Input: part model. Units: mm. Frame: model coordinates. Face numbers are marked on the shaded views. A direction names the side the tool comes from. Give positions to 0.01 mm unless a question says otherwise; leave off trailing zeros. Order: outer loops, then holes, each group sorted by start corner. A loop starts at its lowest first (then second) coordinate and runs counter-clockwise, first axis right, second up. Notation, with made-up numbers: M -32,58 L -12,58 A27 cw -12,90 Z; hole C -11,68 d2. An arc over 180 degrees is marked long. Use a Markdown table: item, result.
from build123d import *

# Parameters (mm, degrees)
CUT_EXTRUDE_1_DEPTH = 3.5


with BuildPart() as part:
    # 草图1 → 旋转1 (revolve)
    with BuildSketch(Plane.XY, mode=Mode.PRIVATE) as revolve_1_sk:
        with BuildLine():
            Line((-108.930747922, 0), (-108.930747922, 13))
            Line((-108.930747922, 13), (-106.930747922, 15))
            Line((-106.930747922, 15), (-80.930747922, 15))
            Line((-80.930747922, 15), (-80.930747922, 20))
            Line((-80.930747922, 20), (-71.930747922, 20))
            Line((-71.930747922, 20), (-71.930747922, 24))
            Line((-71.930747922, 24), (-69.930747922, 26))
            Line((-69.930747922, 26), (-15.930747922, 26))
            Line((-15.930747922, 26), (-13.930747922, 24))
            Line((-13.930747922, 24), (-13.930747922, 20))
            Line((-13.930747922, 20), (-4.930747922, 20))
            Line((-4.930747922, 20), (-4.930747922, 15))
            Line((-4.930747922, 15), (23.069252078, 15))
            Line((23.069252078, 15), (23.069252078, 14))
            ThreePointArc((23.069252078, 14), (23.508591906, 12.939339828), (24.569252078, 12.5))
            Line((24.569252078, 12.5), (81.069252078, 12.5))
            Line((81.069252078, 12.5), (81.069252078, 11.5))
            ThreePointArc((81.069252078, 11.5), (81.508591906, 10.439339828), (82.569252078, 10))
            Line((82.569252078, 10), (115.069252078, 10))
            Line((115.069252078, 10), (117.069252078, 8))
            Line((117.069252078, 8), (117.069252078, 0))
            Line((117.069252078, 0), (-108.930747922, 0))
        make_face()
    revolve(revolve_1_sk.sketch.rotate(Axis((-108.930747922, 0, 0), (1, 0, 0)), 90), axis=Axis((-108.930747922, 0, 0), (1, 0, 0)))

    # 草图2 → 切除-拉伸1 (cut)
    with BuildSketch(Plane(origin=(0, 0, -10), x_dir=(-1, 0, 0), z_dir=(0, 0, -1))):
        with BuildLine():
            Line((-110.808670822, 3), (-88.808670822, 3))
            ThreePointArc((-88.808670822, 3), (-85.808670822, 0), (-88.808670822, -3))
            Line((-88.808670822, -3), (-110.808670822, -3))
            ThreePointArc((-110.808670822, -3), (-113.808670822, 0), (-110.808670822, 3))
        make_face()
    extrude(amount=-CUT_EXTRUDE_1_DEPTH, mode=Mode.SUBTRACT)


solid = part.part
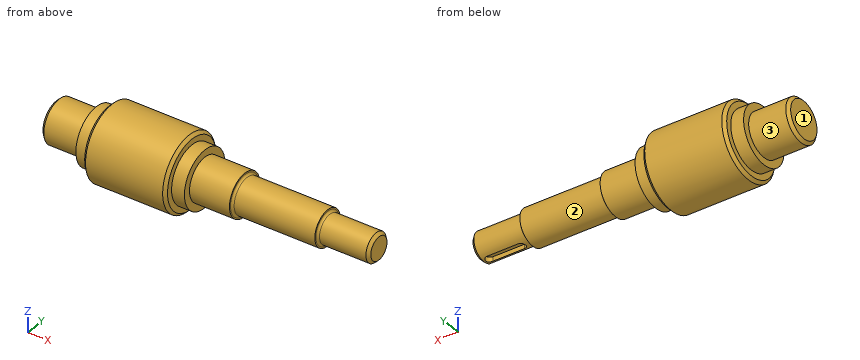
1) Cut plane C-C on x = 2.5. Return loops of the section in (y, z), and give its area (3 significant figures).
Response values:
| item | result |
|---|---|
| outline | C 0,0 d30 |
| area | 707 mm² |
2) Cut plane A-A on x = 47.5. Return loops of the section in (y, z).
Response values:
| item | result |
|---|---|
| outline | C 0,0 d25 |
3) First-contact query: pin 1 Ø1.5 at (y, z) = (-9, 17.5) entering from +X; pin 2 Ø1 at (y, z) = (-9.5, 16) entering from -X; pin 3 Ø1.5 at (x, z) = (95, -7.5) entering from -Y; pin 4 Ø14.5 at (y, z) = (-5.5, 11.5) entering from +X. Flat tips, straight axial feed; report the tip coordinate or a pass-through.
Response values:
| item | result |
|---|---|
| pin 1 | stops at x = -4.93 |
| pin 2 | stops at x = -80.93 |
| pin 3 | stops at y = -7.38 |
| pin 4 | stops at x = 117.07 |
4) Cut plane B-B on x = 101. Return loops of the section in (y, z).
Response values:
| item | result |
|---|---|
| outline | M -3,-9.54 L -3,-6.5 L 3,-6.5 L 3,-9.54 A10 ccw long Z |
5) Reachability of the marked faces 1, 2 and 3 from +Z, -Z, +X, -X, +Y, -Y: full face, straight path, thin tool, end or side. Return the list, or none.
Response values:
| item | result |
|---|---|
| face 1 | +Z, -Z, -X, +Y, -Y |
| face 2 | +X |
| face 3 | -X |
6) Material intervals for line 1 (Y direction, x = -21, z = 0.5); line 2 (Y direction, x = -91, z = 0.5); line 3 (Z direction, x = 46, y = -5), sorted ascending. Write a range as from..to.
Response values:
| item | result |
|---|---|
| line 1 | y = -26..26 |
| line 2 | y = -14.99..14.99 |
| line 3 | z = -11.46..11.46 |
